Input: part model. Units: mm. Frame: model coordinates. A direction names the side the tool comes from. Give positions to 0.01 mm unless a question says otherwise; leave off trailing zeros. Write each loop counter-clockwise with the first axis right and the second up, starting at its lowest first coordinate (ties: lowest second). Pieces come first, ordered by that corner, then holes. Notation, with made-up numbers: (58.25, -6.75) -> (86.25, -6.75) arc R26 ccw to (86.25, 11.25) -> close; hole circle Ø4 at (-39, 71). An arc over 180 degrees is marked (long way). Return JSON: item names as keys, results as strings. Group by question number.
Item 1: Mould query, pull axis Z, two halves, no side actions, for faces 1 (the face through (-9, 149.86, -40)), 2 (the face through (-5, 99, -61)), 3 (the face through (78, 77, 0)). Classes: released by +Z, released by -Z, zero draft, split by the parting line, or undercut.
Item 2: Section C-C, the plane y = 68.5. Return loops of the section in (x, z).
Item 3: Pin query (flat end, axial travel): P1, Ø0.8, axis at x = 1, z = -19.5, coming from the -Y side; P2, Ø6, axis at y = 100, z = -64, coming from the -X side; P3, Ø4.5, axis at x = -12.7, z = -12.7, coming from the -Y side. Return the tip coordinate at first contact, or that it passes through.
Item 4: Section B-B, the plane z = -76. Return loops of the section in (x, y), then the cut area to 3 significant figures.
Item 5: Set-up query: faces 4 (the face through (88, 41, -12.7)), 5 (the face through (99.076, 47.741, -74.841)), 6 (the face through (100, 158, -27.94)). Return all of +Z, -Z, +X, -X, +Y, -Y with unobstructed straight access to the full face (end or side cutting, diameter ignored); none if empty.
Item 6: Section D-D, the plane y = 101.6. Count the separate pieces of the cut face and the enclosed holes in it, then the cut area to 3 significant figures.
Item 7: Line query: line 1 (Y direction, x = 83, z = -19.05); line 2 (X direction, y = 33, z = -61.5); line 3 (Z direction, x = 67.5, y = 129). Output: solid intervals per line, ascending. Write a range as [from, to].
Item 8: Section A-A, the plane x = 136. Return loops of the section in (y, z).
from build123d import *

# Parameters (mm, degrees)
SKETCH1_W            = 81.28
SKETCH1_H            = 81.28
SKETCH1_W_2          = 76.2
SKETCH1_H_2          = 76.2
BOSS_EXTRUDE1_DEPTH  = 177.8
SKETCH2_W            = 2.54
SKETCH2_H            = 38.1
BOSS_EXTRUDE2_DEPTH  = 25.4
SKETCH3_W            = 2.54
SKETCH3_H            = 25.4
CUT_EXTRUDE1_DEPTH   = 212.720846399
BOSS_EXTRUDE3_DEPTH  = 12.7
BOSS_EXTRUDE4_DEPTH  = 12.7
SKETCH14_W           = 5.08
SKETCH14_H           = 25.4
BOSS_EXTRUDE6_DEPTH  = 76.2
CUT_EXTRUDE2_REACH   = 243.407
SKETCH16_W           = 24.13
SKETCH16_H           = 20.32
SKETCH22_R           = 2
CUT_EXTRUDE6_DEPTH   = 252.036309724
SKETCH28_W           = 25.4
SKETCH28_H           = 50.8
BOSS_EXTRUDE7_DEPTH  = 38.1
CUT_EXTRUDE8_REACH   = 245.43
SKETCH32_W           = 33.02
SKETCH32_H           = 20.32
CUT_EXTRUDE9_DEPTH   = 25.4
CUT_EXTRUDE13_REACH  = 245.27
SKETCH34_R           = 8.89
BOSS_EXTRUDE9_DEPTH  = 2.54
SKETCH38_W           = 2.54
SKETCH38_H           = 25.4
CUT_EXTRUDE15_DEPTH  = 63.5
CUT_EXTRUDE17_REACH  = 224.71
SKETCH40_R           = 2.5
BOSS_EXTRUDE10_START = 5
SKETCH41_R           = 3.77
SKETCH41_R_2         = 2.5
BOSS_EXTRUDE10_DEPTH = 5
SKETCH42_R           = 3.77
SKETCH42_R_2         = 2.5
BOSS_EXTRUDE11_DEPTH = 5
SKETCH43_W           = 76.2
SKETCH43_H           = 76.2
CUT_EXTRUDE20_DEPTH  = 25.4
SKETCH44_W           = 174.6
SKETCH44_H           = 70
SKETCH44_R           = 1.5
BOSS_EXTRUDE12_DEPTH = 2.54
BOSS_EXTRUDE13_DEPTH = 2.54
BOSS_EXTRUDE14_DEPTH = 2.54
BOSS_EXTRUDE15_REACH = 264.115
BOSS_EXTRUDE16_DEPTH = 2.54
BOSS_EXTRUDE17_DEPTH = 2.54
BOSS_EXTRUDE18_REACH = 264.115
SKETCH51_R           = 2
CUT_EXTRUDE21_DEPTH  = 2.54
FILLET1_R            = 5.08
FILLET2_R            = 12.7
FILLET3_R            = 2.54
FILLET4_R            = 2.54
FILLET5_R            = 2.54
FILLET7_R            = 12.7
FILLET9_R            = 12.7


with BuildPart() as part:
    # Sketch1 → Boss-Extrude1 (new body)
    with BuildSketch(Plane(origin=(0, 0, 0), x_dir=(1, 0, 0), z_dir=(0, 1, 0))):
        with Locations((40.64, 40.64)):
            Rectangle(SKETCH1_W, SKETCH1_H)
        with Locations((40.64, 40.64)):
            Rectangle(SKETCH1_W_2, SKETCH1_H_2, mode=Mode.SUBTRACT)
    extrude(amount=BOSS_EXTRUDE1_DEPTH)

    # Sketch2 → Boss-Extrude2 (add)
    with BuildSketch(Plane(origin=(0, 0, 0), x_dir=(0, 0, -1), z_dir=(1, 0, 0))):
        with Locations((64.77, 19.05)):
            Rectangle(SKETCH2_W, SKETCH2_H)
    extrude(amount=-BOSS_EXTRUDE2_DEPTH)

    # Sketch3 → Cut-Extrude1 (cut, through all)
    with BuildSketch(Plane.XY):
        with Locations((80.01, 12.7)):
            Rectangle(SKETCH3_W, SKETCH3_H)
    extrude(amount=-CUT_EXTRUDE1_DEPTH, mode=Mode.SUBTRACT)

    # Sketch7 → Boss-Extrude3 (add)
    with BuildSketch(Plane.XY):
        Polygon((81.28, 25.4), (106.68, 50.8), (81.28, 50.8), align=None)
    extrude(amount=-BOSS_EXTRUDE3_DEPTH)

    # Sketch10 → Boss-Extrude4 (add)
    with BuildSketch(Plane(origin=(0, 0, -81.28), x_dir=(-1, 0, 0), z_dir=(0, 0, -1))):
        Polygon((-81.28, 25.4), (-81.28, 50.8), (-106.68, 50.8), align=None)
    extrude(amount=-BOSS_EXTRUDE4_DEPTH)

    # Sketch14 → Boss-Extrude6 (add)
    with BuildSketch(Plane(origin=(81.28, 0, 0), x_dir=(0, 0, -1), z_dir=(1, 0, 0))):
        with Locations((40.64, 38.1)):
            Rectangle(SKETCH14_W, SKETCH14_H)
    extrude(amount=BOSS_EXTRUDE6_DEPTH)

    # Sketch16 → Cut-Extrude2 (cut, up to next)
    with BuildSketch(Plane.XY.offset(-38.1), mode=Mode.PRIVATE) as cut_extrude2_sk1:
        with Locations((128.905, 40.64)):
            Rectangle(SKETCH16_W, SKETCH16_H)
    cut_extrude2_tool1 = extrude(cut_extrude2_sk1.sketch, amount=-CUT_EXTRUDE2_REACH, mode=Mode.PRIVATE) & part.part
    add(cut_extrude2_tool1.solids().sort_by_distance((128.905, 40.64, -38.1))[0], mode=Mode.SUBTRACT)

    # Sketch22 → Cut-Extrude6 (cut, through all)
    with BuildSketch(Plane.XY):
        with Locations((93.98, 45.72)):
            Circle(SKETCH22_R)
    extrude(amount=-CUT_EXTRUDE6_DEPTH, mode=Mode.SUBTRACT)

    # Sketch28 → Boss-Extrude7 (add)
    with BuildSketch(Plane(origin=(81.28, 0, 0), x_dir=(0, 0, -1), z_dir=(1, 0, 0))):
        with Locations((40.64, 152.4)):
            Rectangle(SKETCH28_W, SKETCH28_H)
    extrude(amount=BOSS_EXTRUDE7_DEPTH)

    # Sketch30 → Cut-Extrude8 (cut, up to next)
    with BuildSketch(Plane.XY.offset(-27.94), mode=Mode.PRIVATE) as cut_extrude8_sk1:
        Polygon((81.28, 127), (119.38, 127), (119.38, 152.4), align=None)
    cut_extrude8_tool1 = extrude(cut_extrude8_sk1.sketch, amount=-CUT_EXTRUDE8_REACH, mode=Mode.PRIVATE) & part.part
    add(cut_extrude8_tool1.solids().sort_by_distance((106.68, 135.466667, -27.94))[0], mode=Mode.SUBTRACT)

    # Sketch32 → Cut-Extrude9 (cut)
    with BuildSketch(Plane(origin=(0, 177.8, 0), x_dir=(1, 0, 0), z_dir=(0, 1, 0))):
        with Locations((100.33, 40.64)):
            Rectangle(SKETCH32_W, SKETCH32_H)
    extrude(amount=-CUT_EXTRUDE9_DEPTH, mode=Mode.SUBTRACT)

    # Cut-Extrude13: up to this face of the body (flat: up to its plane)
    cut_extrude13_end = Plane(part.part.faces().sort_by_distance((78.74, 101.6, -40.64))[0])
    # Sketch34 → Cut-Extrude13 (cut, up to the picked face)
    with BuildSketch(Plane(origin=(119.38, 0, 0), x_dir=(0, 0, -1), z_dir=(1, 0, 0)), mode=Mode.PRIVATE) as cut_extrude13_sk1:
        with Locations(Location((40.64, 165.1, 0), (0, 0, 180))):
            Circle(SKETCH34_R)
    cut_extrude13_tool1 = split(extrude(cut_extrude13_sk1.sketch, amount=-CUT_EXTRUDE13_REACH, mode=Mode.PRIVATE), bisect_by=cut_extrude13_end, keep=Keep.BOTH, mode=Mode.PRIVATE)
    add(cut_extrude13_tool1.solids().sort_by(Axis((119.38, 165.1, -40.64), (-1, 0, 0)))[0], mode=Mode.SUBTRACT)

    # Sketch37 → Boss-Extrude9 (add)
    with BuildSketch(Plane.XY.offset(-63.5)):
        Polygon((-25.4, 38.1), (0, 38.1), (0, 52.764696837), align=None)
    extrude(amount=-BOSS_EXTRUDE9_DEPTH)

    # Sketch38 → Cut-Extrude15 (cut)
    with BuildSketch(Plane.XY):
        with Locations((1.27, 12.7)):
            Rectangle(SKETCH38_W, SKETCH38_H)
    extrude(amount=-CUT_EXTRUDE15_DEPTH, mode=Mode.SUBTRACT)

    # Cut-Extrude17: up to this face of the body (flat: up to its plane)
    cut_extrude17_end = Plane(part.part.faces().sort_by_distance((0, 99.23335202, -41.514066738))[0])
    # Sketch40 → Cut-Extrude17 (cut, up to the picked face)
    with BuildSketch(Plane(origin=(81.28, 0, 0), x_dir=(0, 0, -1), z_dir=(1, 0, 0)), mode=Mode.PRIVATE) as cut_extrude17_sk1:
        with Locations((19.05, 101.6)):
            Circle(SKETCH40_R)
    cut_extrude17_tool1 = split(extrude(cut_extrude17_sk1.sketch, amount=-CUT_EXTRUDE17_REACH, mode=Mode.PRIVATE), bisect_by=cut_extrude17_end, keep=Keep.BOTH, mode=Mode.PRIVATE)
    # Sketch40 → Cut-Extrude17 (cut, up to the picked face)
    with BuildSketch(Plane(origin=(81.28, 0, 0), x_dir=(0, 0, -1), z_dir=(1, 0, 0)), mode=Mode.PRIVATE) as cut_extrude17_sk2:
        with Locations((62.23, 101.6)):
            Circle(SKETCH40_R)
    cut_extrude17_tool2 = split(extrude(cut_extrude17_sk2.sketch, amount=-CUT_EXTRUDE17_REACH, mode=Mode.PRIVATE), bisect_by=cut_extrude17_end, keep=Keep.BOTH, mode=Mode.PRIVATE)
    add(cut_extrude17_tool1.solids().sort_by(Axis((81.28, 101.6, -19.05), (-1, 0, 0)))[0], mode=Mode.SUBTRACT)
    add(cut_extrude17_tool2.solids().sort_by(Axis((81.28, 101.6, -62.23), (-1, 0, 0)))[0], mode=Mode.SUBTRACT)

    # Sketch41 → Boss-Extrude10 (add)
    # profile 1 of 2: a face of its own
    with BuildSketch(Plane(origin=(81.28, 0, 0), x_dir=(0, 0, -1), z_dir=(1, 0, 0)).offset(BOSS_EXTRUDE10_START)):
        with Locations(Location((19.05, 101.6, 0), (0, 0, 180))):
            Circle(SKETCH41_R)
        with Locations((19.05, 101.6)):
            Circle(SKETCH41_R_2, mode=Mode.SUBTRACT)
    # profile 2 of 2: a face of its own
    with BuildSketch(Plane(origin=(81.28, 0, 0), x_dir=(0, 0, -1), z_dir=(1, 0, 0)).offset(BOSS_EXTRUDE10_START)):
        with Locations(Location((62.23, 101.6, 0), (0, 0, 180))):
            Circle(SKETCH41_R)
        with Locations((62.23, 101.6)):
            Circle(SKETCH41_R_2, mode=Mode.SUBTRACT)
    extrude(amount=-BOSS_EXTRUDE10_DEPTH)

    # Sketch42 → Boss-Extrude11 (add)
    # profile 1 of 2: a face of its own
    with BuildSketch(Plane.ZY):
        with Locations((-62.23, 101.6)):
            Circle(SKETCH42_R)
        with Locations(Location((-62.23, 101.6, 0), (0, 0, 180))):
            Circle(SKETCH42_R_2, mode=Mode.SUBTRACT)
    # profile 2 of 2: a face of its own
    with BuildSketch(Plane.ZY):
        with Locations((-19.05, 101.6)):
            Circle(SKETCH42_R)
        with Locations(Location((-19.05, 101.6, 0), (0, 0, 180))):
            Circle(SKETCH42_R_2, mode=Mode.SUBTRACT)
    extrude(amount=BOSS_EXTRUDE11_DEPTH)

    # Sketch43 → Cut-Extrude20 (cut)
    with BuildSketch(Plane(origin=(0, 177.8, 0), x_dir=(1, 0, 0), z_dir=(0, 1, 0))):
        Polygon((83.82, 53.34), (83.82, 27.94), (81.28, 27.94), (81.28, 0), (0, 0), (0, 81.28), (81.28, 81.28), (81.28, 53.34), align=None)
        with Locations((40.64, 40.64)):
            Rectangle(SKETCH43_W, SKETCH43_H, mode=Mode.SUBTRACT)
    extrude(amount=-CUT_EXTRUDE20_DEPTH, mode=Mode.SUBTRACT)

    # Sketch44 → Boss-Extrude12 (add)
    with BuildSketch(Plane.XY):
        with Locations((87.3, 85.8)):
            Rectangle(SKETCH44_W, SKETCH44_H)
        with Locations((140.97, 115.8)):
            Circle(SKETCH44_R, mode=Mode.SUBTRACT)
        with Locations((140.97, 55.8)):
            Circle(SKETCH44_R, mode=Mode.SUBTRACT)
    extrude(amount=-BOSS_EXTRUDE12_DEPTH)

    # Sketch45 → Boss-Extrude13 (add)
    with BuildSketch(Plane.XY):
        Polygon((0, 152.4), (-25.4, 152.4), (0, 127), align=None)
    extrude(amount=-BOSS_EXTRUDE13_DEPTH)

    # Sketch46 → Boss-Extrude14 (add)
    with BuildSketch(Plane(origin=(0, 0, -81.28), x_dir=(-1, 0, 0), z_dir=(0, 0, -1))):
        Polygon((0, 152.4), (0, 127), (25.4, 152.4), align=None)
    extrude(amount=-BOSS_EXTRUDE14_DEPTH)

    # Sketch47 → Boss-Extrude15 (add, up to next)
    with BuildSketch(Plane.XY, mode=Mode.PRIVATE) as boss_extrude15_sk1:
        Polygon((0, 152.4), (-25.4, 152.4), (-22.86, 149.86), (0, 149.86), align=None)
    boss_extrude15_tool1 = extrude(boss_extrude15_sk1.sketch, amount=-BOSS_EXTRUDE15_REACH, mode=Mode.PRIVATE) - part.part
    add(boss_extrude15_tool1.solids().sort_by_distance((-12.07614, 151.152281, 0))[0])

    # Sketch48 → Boss-Extrude16 (add)
    with BuildSketch(Plane.XY):
        Polygon((81.28, 152.4), (106.68, 152.4), (81.28, 127), align=None)
    extrude(amount=-BOSS_EXTRUDE16_DEPTH)

    # Sketch49 → Boss-Extrude17 (add)
    with BuildSketch(Plane(origin=(0, 0, -81.28), x_dir=(-1, 0, 0), z_dir=(0, 0, -1))):
        Polygon((-81.28, 152.4), (-106.68, 152.4), (-81.28, 127), align=None)
    extrude(amount=-BOSS_EXTRUDE17_DEPTH)

    # Sketch50 → Boss-Extrude18 (add, up to next)
    with BuildSketch(Plane(origin=(0, 0, -81.28), x_dir=(-1, 0, 0), z_dir=(0, 0, -1)), mode=Mode.PRIVATE) as boss_extrude18_sk1:
        Polygon((-81.28, 152.4), (-106.68, 152.4), (-104.14, 149.86), (-81.28, 149.86), align=None)
    boss_extrude18_tool1 = extrude(boss_extrude18_sk1.sketch, amount=-BOSS_EXTRUDE18_REACH, mode=Mode.PRIVATE) - part.part
    add(boss_extrude18_tool1.solids().sort_by_distance((93.35614, 151.152281, -81.28))[0])
    add(boss_extrude18_tool1.solids().sort_by_distance((93.35614, 151.152281, -81.28))[1])

    # Sketch51 → Cut-Extrude21 (cut)
    with BuildSketch(Plane(origin=(0, 152.4, 0), x_dir=(1, 0, 0), z_dir=(0, 1, 0))):
        with Locations(Location((-12.7, 68.58, 0), (0, 0, 270))):
            Circle(SKETCH51_R)
        with Locations(Location((-12.7, 40.64, 0), (0, 0, 270))):
            Circle(SKETCH51_R)
        with Locations(Location((-12.7, 12.7, 0), (0, 0, 270))):
            Circle(SKETCH51_R)
        with Locations(Location((93.98, 68.58, 0), (0, 0, 270))):
            Circle(SKETCH51_R)
        with Locations(Location((93.98, 12.7, 0), (0, 0, 270))):
            Circle(SKETCH51_R)
    extrude(amount=-CUT_EXTRUDE21_DEPTH, mode=Mode.SUBTRACT)

    # Fillet1
    fillet1_edges = [part.edges().sort_by_distance(p)[0] for p in [
        (106.68, 50.8, -7.62),
        (106.68, 50.8, -74.93),
    ]]
    fillet(fillet1_edges, radius=FILLET1_R)

    # Fillet2
    fillet2_edges = [part.edges().sort_by_distance(p)[0] for p in [
        (174.6, 120.8, -1.27),
        (174.6, 50.8, -1.27),
    ]]
    fillet(fillet2_edges, radius=FILLET2_R)

    # Fillet3
    fillet3_edges = [part.edges().sort_by_distance(p)[0] for p in [
        (157.48, 50.8, -40.64),
        (157.48, 25.4, -40.64),
    ]]
    fillet(fillet3_edges, radius=FILLET3_R)

    # Fillet4
    # the kernel refuses this fillet: 2.54 mm, written as the material it takes off along each edge
    with BuildSketch(Plane(origin=(-25.4, 152.4, 15.330256121), x_dir=(1, 0, 0), z_dir=(0, 0, -1))) as fillet4_piece_1:
        with BuildLine():
            CenterArc((FILLET4_R * 2.41421356237, FILLET4_R), FILLET4_R, 135, 135)
            Line((FILLET4_R * 1.70710678119, FILLET4_R * 1.70710678119), (0, 0))
            Line((0, 0), (FILLET4_R * 2.41421356237, 0))
        make_face()
    extrude(amount=111.940512242, mode=Mode.SUBTRACT)

    # Fillet5
    fillet5_edges = [part.edges().sort_by_distance(p)[0] for p in [
        (106.68, 152.4, -67.31),
        (106.68, 152.4, -13.97),
    ]]
    fillet(fillet5_edges, radius=FILLET5_R)

    # Fillet7
    fillet7_edges = [part.edges().sort_by_distance(p)[0] for p in [
        (-25.4, 38.1, -64.77),
    ]]
    fillet(fillet7_edges, radius=FILLET7_R)

    # Fillet9
    fillet9_edges = [part.edges().sort_by_distance(p)[0] for p in [
        (83.82, 177.8, -29.21),
        (83.82, 177.8, -52.07),
    ]]
    fillet(fillet9_edges, radius=FILLET9_R)


solid = part.part
Answer below:
{
 "1": {"face 1": "undercut", "face 2": "zero draft", "face 3": "released by +Z"},
 "2": {"outline": "(0, -81.28) -> (81.28, -81.28) -> (81.28, -2.54) -> (174.6, -2.54) -> (174.6, 0) -> (0, 0) -> close; hole (2.54, -78.74) -> (78.74, -78.74) -> (78.74, -2.54) -> (2.54, -2.54) -> close"},
 "3": {"P1": "stops at y = 25.4", "P2": "stops at x = -5", "P3": "stops at y = 149.86"},
 "4": {"outline": "(-21.81, 149.86) -> (0, 149.86) -> (0, 0) -> (2.54, 0) -> (2.54, 152.4) -> (-19.27, 152.4) arc R2.54 ccw to start; (78.74, 25.4) -> (81.28, 25.4) -> (98.01, 42.13) arc R5.08 ccw to (94.42, 50.8) -> (81.28, 50.8) -> (81.28, 149.86) -> (103.09, 149.86) arc R2.54 ccw to (100.55, 152.4) -> (78.74, 152.4) -> close; hole circle Ø4 at (93.98, 45.72)", "area": "1,100 mm2"},
 "5": {"face 4": "+X, -Y", "face 5": "-Z, +X", "face 6": "+X"},
 "6": {"separate pieces": "4", "enclosed holes": "0", "area": "1,040 mm2"},
 "7": {"line 1": "y = [97.83, 99.1], [104.1, 105.37], [149.86, 152.4]", "line 2": "x = [0, 2.54], [78.74, 81.28]", "line 3": "z = [-81.28, -78.74], [-2.54, 0]"},
 "8": {"outline": "(25.4, -43.18) -> (30.48, -43.18) -> (30.48, -38.1) -> (25.4, -38.1) -> close; (50.8, -2.54) -> (120.8, -2.54) -> (120.8, 0) -> (50.8, 0) -> close"}
}
